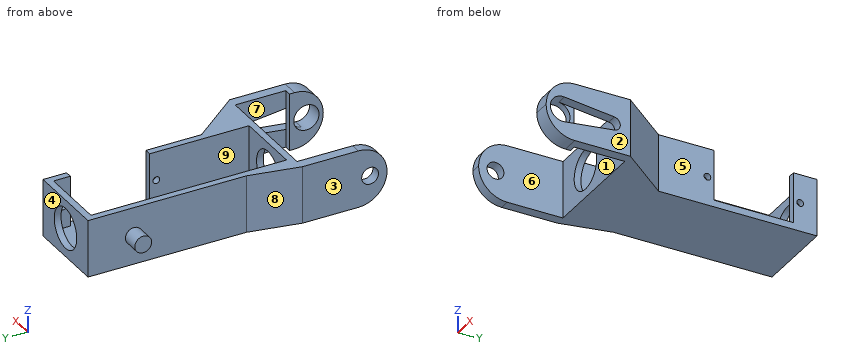
Autodesk Inventor part; units mm, degrees
ref_plane "YZ Plane" through (0, 0, 0) normal (1, 0, 0) x (0, 1, 0)
ref_plane "XZ Plane" through (0, 0, 0) normal (0, 1, 0) x (-1, 0, 0)
ref_plane "XY Plane" through (0, 0, 0) normal (0, 0, 1) x (1, 0, 0)
sketch "Sketch1" plane through (0, 0, 0) normal (0, 0, 1) x (1, 0, 0)
  line L0 (0, 0) -> (24, 0)
  line L1 (24, 0) -> (24, -60)
  line L2 (24, -60) -> (0, -60)
  line L3 (0, -60) -> (0, 0)
  dimension "d0" = 24
  dimension "d1" = 60
extrude "Extrusion1" add sketch "Sketch1" along normal blind 2
sketch "Sketch2" plane through (0, 0, 2) normal (0, 0, 1) x (1, 0, 0)
  line L0 (0, -60) -> (24, -60)
  line L1 (0, 0) -> (2, 0)
  line L2 (2, 0) -> (2, -60)
  line L3 (2, -60) -> (0, -60)
  line L4 (0, -60) -> (0, 0)
  line L5 (24, -60) -> (24, 0)
  line L6 (24, 0) -> (22, 0)
  line L7 (22, 0) -> (22, -60)
  line L8 (22, -60) -> (24, -60)
  line L9 (24, -60) -> (24, 0)
  dimension "d4" = 2
  dimension "d5" = 2
extrude "Extrusion2" add sketch "Sketch2" along normal blind 15
sketch "Sketch3" plane through (24, -60, 0) normal (1, 0, 0) x (0, 0, -1)
  circle A0 centre (-8.5, 57) radius 1
  circle A1 centre (-8.5, 29.5) radius 1
  line L0 (-17, 0) -> (-17, 60)
  line L1 (0, 60) -> (-17, 60)
  dimension "d8" = 2
  dimension "d9" = 2
  dimension "d10" = 8.5
  dimension "d11" = 8.5
  dimension "d12" = 27.5
  dimension "d13" = 3
extrude "Extrusion3" cut sketch "Sketch3" against normal up to surface (2 mm away)
sketch "Sketch4" plane through (24, -60, 0) normal (1, 0, 0) x (0, 0, -1)
  line L0 (-17, 60) -> (-17, 0)
  line L1 (-17, 55) -> (-2, 55)
  line L2 (-2, 55) -> (-2, 31.5)
  line L3 (-2, 31.5) -> (-17, 31.5)
  line L4 (-17, 31.5) -> (-17, 55)
  circle A0 centre (-8.5, 57) radius 1
  circle A1 centre (-8.5, 29.5) radius 1
  point P0 (-17, 31.5)
  dimension "d23" = 15
  dimension "d24" = 23.5
  dimension "d25" = 2
  dimension "d26" = 2
extrude "Extrusion4" cut sketch "Sketch4" against normal up to surface (2 mm away) contours L1 L2 L3 L0
sketch "Sketch5" plane through (0, -60, 0) normal (-1, 0, 0) x (0, 0, 1)
  circle A0 centre (8.5, 48.4) radius 2.5
  circle A1 centre (8.5, 57) radius 1
  point P0 (0, 60)
  dimension "d29" = 5
  dimension "d32" = 8.6
  dimension "d33" = 0
extrude "Extrusion5" add sketch "Sketch5" along normal blind 5 contours A0
sketch "Sketch12" plane through (0, 0, 0) normal (0, 0, -1) x (-1, 0, 0)
  line L0 (3, -60) -> (-36, -60)
  line L1 (-36, -60) -> (-36, -85)
  line L2 (-36, -85) -> (3, -85)
  line L3 (3, -85) -> (3, -60)
  line L4 (0, 0) -> (0, -60)
  line L5 (-2, -60) -> (-22, -60)
  line L6 (3, -60) -> (0, -60)
  line L7 (0, -60) -> (0, -85)
  line L8 (0, -85) -> (3, -85)
  line L9 (3, -85) -> (3, -60)
  line L10 (-36, -60) -> (-31, -60)
  line L11 (-31, -60) -> (-31, -85)
  line L12 (-31, -85) -> (-36, -85)
  line L13 (-36, -85) -> (-36, -60)
  line L14 (-31, -60) -> (-33, -60)
  line L15 (-33, -60) -> (-33, -75)
  line L16 (-33, -75) -> (-31, -75)
  line L17 (-31, -75) -> (-31, -60)
  dimension "d52" = 3
  dimension "d53" = 25
  dimension "d54" = 0
  dimension "d55" = 3
  dimension "d56" = 5
  dimension "d83" = 31
  dimension "d92" = 2
  dimension "d93" = 15
extrude "Extrusion9" add sketch "Sketch12" against normal up to surface (17 mm away) contours L3 L2 L7 L0 | L2 L1 L0 L15 L16 L11
sketch "Sketch13" plane through (0, 0, 0) normal (0, 0, -1) x (-1, 0, 0)
  line L0 (-33, -60) -> (-36, -60)
  line L1 (0, -60) -> (-24, -60)
  line L2 (-36, -60) -> (-24, -60)
  line L3 (-24, -60) -> (-24, -45)
  line L4 (-24, -45) -> (-36, -60)
  line L5 (0, -60) -> (0, -45)
  line L6 (0, 0) -> (0, -60)
  line L7 (0, -60) -> (15, -60) construction
  line L8 (0, -45) -> (3, -60)
  line L9 (3, -60) -> (0, -60)
  point P0 (-31, -60)
  dimension "d59" = 15
  dimension "d60" = 90
  dimension "d63" = 15
  dimension "d64" = 90
extrude "Extrusion10" add sketch "Sketch13" against normal up to surface (17 mm away)
sketch "Sketch14" plane through (-3, -85, 0) normal (-1, 0, 0) x (0, 0, 1)
  circle A0 centre (8.5, 5) radius 2.5
  line L0 (17, 0) -> (17, 25)
  line L1 (0, 25) -> (17, 25)
  point P0 (0, 85)
  dimension "d65" = 5
  dimension "d66" = 8.5
  dimension "d67" = 20
extrude "Extrusion11" cut sketch "Sketch14" against normal up to surface (39 mm away)
sketch "Sketch15" plane through (0, 0, 0) normal (0, 1, 0) x (1, 0, 0)
  line L0 (24, -17) -> (24, 0)
  line L1 (2, -17) -> (0, -17)
  line L2 (24, 0) -> (0, 0)
  line L3 (0, 0) -> (0, -17)
  line L4 (0, -17) -> (24, -17)
  line L5 (24, -17) -> (24, 0)
extrude "Extrusion12" add sketch "Sketch15" along normal blind 2
sketch "Sketch16" plane through (2, -60, 2) normal (0, -1, 0) x (1, 0, 0)
  line L0 (0, 15) -> (20, 15)
  line L1 (0, 0) -> (20, 0)
  line L2 (0, 15) -> (20, 15)
  line L3 (20, 15) -> (20, 0)
  line L4 (20, 0) -> (0, 0)
  line L5 (0, 0) -> (0, 15)
  point P0 (-2, -2)
  point P1 (20, 15)
extrude "Extrusion13" add sketch "Sketch16" against normal blind 2
sketch "Sketch17" plane through (0, 2, 0) normal (0, 1, 0) x (1, 0, 0)
  circle A0 centre (12, -8.5) radius 6
  line L0 (24, -17) -> (24, 0)
  line L1 (24, 0) -> (0, 0)
  dimension "d74" = 12
  dimension "d75" = 12
  dimension "d76" = 8.5
extrude "Extrusion14" cut sketch "Sketch17" against normal up to surface (62 mm away)
fillet "Fillet2" radius 8.5 4 edges at (33.5, -85, 0) (-1.5, -85, 0) (33.5, -85, 17) (-1.5, -85, 17)
sketch "Sketch18" plane through (36, -60, 17) normal (1, 0, 0) x (0, 0, -1)
  circle A0 centre (8.5, -20) radius 2.5
  circle A1 centre (8.5, -20) radius 3.75
  point P0 (17, 60)
  dimension "d80" = 7.5
extrude "Extrusion15" cut sketch "Sketch18" against normal up to surface (5 mm away) contours A0 | A1
sketch "Sketch20" plane through (36, -60, 17) normal (1, 0, 0) x (0, 0, -1)
  circle A0 centre (8.5, -5) radius 2
  circle A1 centre (8.5, -20) radius 3.75
  line L0 (10.4863, -4.7667) -> (12.2244, -19.5625)
  line L1 (6.5137, -4.7667) -> (4.7756, -19.5625)
  circle A2 centre (8.5, -5) radius 2
  circle A3 centre (8.5, -20) radius 3.75
  line L2 (10.4863, -4.7667) -> (12.2244, -19.5625)
  line L3 (6.5137, -4.7667) -> (4.7756, -19.5625)
  point P0 (17, 60)
  dimension "d84" = 4
  dimension "d85" = 15
  dimension "d86" = 0
  dimension "d89" = 4
  dimension "d90" = 15
  dimension "d91" = 0
extrude "Extrusion16" cut sketch "Sketch20" against normal blind 3 contours A0 | A0 L0 A1 L1
properties part number "juncao2"
The listing builds one solid part. Answer for the finished solid, in the listing's coordinates (mm). Face numbers are marked on the shaded views. A direction names the side the tool comes from. Give positions to 0.01 mm unless a question says otherwise; leave off trailing zeros. Loops run counter-clockwise (first coordinate to the right, second up) from the corner with the lowest first, then second, coordinate; pieces in that order, holes last. Notation, with made-up numbers: M -4.5,-36.5 L 30.5,-36.5 A22 cw 30.5,-9.5 Z; hole C 82.25,76.5 d6. An arc over 180 degrees is marked long. One line per item, written item: value.
1. Section A-A on x = -1 is taken. State how many separate pieces and enclosed holes the cut face has, plus the area to 3 significant figures.
Found:
separate pieces: 2
enclosed holes: 1
area: 564 mm^2
2. Each of these flat-tipped pins is pushed along its axis until it touches: P1, Ø4, axis at x = 17.5, y = -45, coming from the +Z side; P2, Ø1.2, axis at y = -30.5, z = 8.5, coming from the +X side; P3, Ø7.5, axis at y = -71, z = 5, coming from the -X side. Where does it stop, or does it pass through?
Found:
P1: z = 2
P2: x = 2
P3: x = -3
3. Section B-B on y = -30.5 is taken. Determine the outline of the cut face in (x, z), plus the area to 3 significant figures.
Found:
outline: M 0,0 L 24,0 L 24,7.5 L 22,7.5 L 22,2 L 2,2 L 2,17 L 0,17 Z; M 22,9.5 L 24,9.5 L 24,17 L 22,17 Z
area: 104 mm^2
4. For a pull along X with two mould halves and no side action, classify the marked faces 1, 2, 3 and 4 as pulls with the +X half, pulls with the -X half, needs draft (parallel to the pull), parting line crosses it, or undercut.
Found:
face 1: undercut
face 2: pulls with the +X half
face 3: pulls with the -X half
face 4: needs draft
5. For the marked faces 5, 6, 7, 8 and 9, determine the directions among +Z, -Z, +X, -X, +Y, -Y from which every point of the face is accessible in a straight line to the end or side of a thin tool.
Found:
face 5: +Z, -Z, +X, +Y
face 6: +Z, -Z, -Y
face 7: +Z, -Z
face 8: +Z, -Z, -X
face 9: +Z
6. Section C-C on x = 12 is taken. Determine the outline of the cut face in (y, z).
Found:
outline: M -60,0 L 2,0 L 2,2.5 L 0,2.5 L 0,2 L -58,2 L -58,2.5 L -60,2.5 Z; M -60,14.5 L -58,14.5 L -58,17 L -60,17 Z; M 0,14.5 L 2,14.5 L 2,17 L 0,17 Z
7. Section D-D on y = -50 is taken. Determine the outline of the cut face in (x, z), plus the area to 3 significant figures.
Found:
outline: M -1,0 L 28,0 L 28,17 L 22,17 L 22,2 L 2,2 L 2,17 L -1,17 Z
area: 193 mm^2
8. Find the intervals of material crossed by probe 1 along Y at (x, z) = (23.2, 8.5); probe 2 along Y at (x, z) = (18, 5.75); probe 3 along X at (y, z) = (-66, 5), in increasing order.
Found:
probe 1: -60 to -31.5, -29.5 to -28.5, -5 to -4, -2 to 2
probe 2: -60 to -58, 0 to 2
probe 3: -3 to 0, 33 to 36
